Autodesk Inventor part; units mm, degrees
sketch "Sketch1" plane through (0, 0, 0) normal (0, 0, 1) x (1, 0, 0)
  line L0 (0, 0) -> (34, 0)
  line L1 (34, 0) -> (34, 4)
  line L2 (34, 4) -> (4, 4)
  line L3 (4, 4) -> (4, 154)
  line L4 (4, 154) -> (0, 154)
  line L5 (0, 154) -> (0, 0)
  dimension "d2" = 34
  dimension "d3" = 4
  dimension "d4" = 30
  dimension "d5" = 150
  dimension "d6" = 4
extrude "Extrusion1" add sketch "Sketch1" along normal blind 34
sketch "Sketch3" plane through (4, 4, 0) normal (1, 0, 0) x (0, 0, -1)
  line L0 (0, 0) -> (-34, 0)
  line L1 (0, 150) -> (-34, 150)
  arc A0 (-27, 20) -> (-7, 20) centre (-17, 20) ccw
  arc A1 (-7, 130) -> (-27, 130) centre (-17, 130) ccw
  line L2 (-27, 20) -> (-27, 130)
  line L3 (-7, 130) -> (-7, 20)
  point P0 (0, -4)
extrude "Extrusion3" cut sketch "Sketch3" against normal blind 20
sketch "Sketch4" plane through (0, 0, 0) normal (0, -1, 0) x (1, 0, 0)
  line L0 (0, 0) -> (34, 0)
  line L1 (34, 0) -> (34, 34)
  line L2 (0, 34) -> (34, 34)
  line L3 (0, 0) -> (0, 34)
  line L4 (4, 34) -> (0, 34)
  line L5 (34, 0) -> (34, 34)
  circle A0 centre (26.9999, 26.9999) radius 1.5
  circle A1 centre (26.9999, 7.0001) radius 1.5
  circle A2 centre (7.0001, 26.9999) radius 1.5
  circle A3 centre (7.0001, 7.0001) radius 1.5
  dimension "d28" = 3
  dimension "d29" = 3
  dimension "d30" = 3
  dimension "d31" = 3
extrude "Extrusion4" cut sketch "Sketch4" against normal blind 10 contours A0 | A1 | A2 | A3
sketch "Sketch5" plane through (4, 4, 0) normal (0, 1, 0) x (1, 0, 0)
  line L0 (0, 0) -> (0, -34)
  line L1 (36.8, 0) -> (-10.8, 0)
  line L2 (30, 0) -> (0, 0)
  line L3 (0, 0) -> (0, -2)
  line L4 (0, 0) -> (0, -34)
  line L5 (0, -2) -> (5, -2)
  line L6 (5, -2) -> (5, 0)
  line L7 (30, -34) -> (0, -34)
  line L8 (0, -34) -> (0, -32)
  line L9 (0, -32) -> (5, -32)
  line L10 (5, -32) -> (5, -34)
  line L11 (5, -34) -> (0, -34)
  point P0 (-4, 0)
  dimension "d34" = 2
  dimension "d35" = 5
  dimension "d36" = 2
  dimension "d37" = 5
extrude "Extrusion5" add sketch "Sketch5" along normal blind 5
sketch "Sketch6" plane through (0, 0, 0) normal (0, 0, -1) x (-1, 0, 0)
  line L0 (-34, 0) -> (-34, 4)
  line L1 (0, 0) -> (-34, 0)
  line L2 (0, 154) -> (0, 0)
  line L3 (-4, 154) -> (0, 154)
  line L4 (-4, 9) -> (-4, 154)
  line L5 (-9, 9) -> (-4, 9)
  line L6 (-9, 4) -> (-9, 9)
  line L7 (-34, 4) -> (-9, 4)
  line L8 (-4, 9) -> (-4, 4)
  line L9 (-9, 4) -> (-4, 9)
  line L10 (-4, 9) -> (-9, 9)
  line L11 (-4, 9) -> (-9, 9)
  line L12 (-9, 4) -> (-9, 9)
  line L13 (-9, 9) -> (-9, 4)
extrude "Extrusion6" cut sketch "Sketch6" against normal blind 4000 contours L6 L5 L9
properties part number "IDOM_infrared_fixture2"
CAD build for the part. Positions are in the model's coordinates, mm. A direction names the side the tool comes from. Round coordinates to 2 decimals unless told otherwise and drop trailing zeros. Write each loop counter-clockwise with the first axis right and the second up, starting at its lowest first coordinate (ties: lowest second). Pieces come first, ordered by that corner, then holes. Notation, with made-up numbers: (71.5, 11) -> (108.5, 11) arc R11 ccw to (108.5, 19) -> close; hole circle Ø1 at (73, 84.25). An arc over 180 degrees is marked (long way). Answer in a Markdown table with one row per item. Add a question column.
Item 1: Saw through at D-D, the plane x = 10.5. Write the cut outline in (y, z), then the cut area to 3 significant figures.
Item 2: Saw through at C-C, the plane z = 23. Write the cut outline in (x, y).
Item 3: Drop flat-ended pins along their axis: pin 1 Ø3.5 at (x, z) = (27, 7) entering from +Y; pin 2 Ø2.5 at (x, y) = (7.5, 7.5) entering from +Z; pin 3 Ø10 at (x, y) = (8, 86) entering from +Z. Give the stop position or say it passes through.
Item 4: Which spindle directions (+Z, -Z, +X, -X, +Y, -Y) get a long thin tool onto all of the face, cutting with end or side? Do faces 1 (the face through (7.806, 1.972, 8.265)), 2 (the face through (2, 78, 27)). Say none if no direction does.
Item 5: Saw through at B-B, the plane y = 87.5. Write the cut outline in (x, z), then the cut area to 3 significant figures.
Item 6: Mould opens along X. For faces 3 (the face through (6, 6, 2)), 4 (the face through (7.806, 1.972, 28.265)), 5 (the face through (4, 78, 28)) say: pulls with the +X half, pulls with the -X half, needs draft (parallel to the pull), parting line crosses it, or undercut.
Item 7: Saw through at A-A, the plane z = 17. Write the cut outline in (x, y), then the cut area to 3 significant figures.
Item 8: Drill centre lines: line 1 (Y direction, x = 23, z = 3); line 2 (Z direction, x = 2, y = 57). Where is each one in solid material? Low to high. Write a range as from..to.
Findings below:
| question | item | result |
|---|---|---|
| 1 | outline | (0, 0) -> (4, 0) -> (4, 34) -> (0, 34) -> close |
| 1 | area | 136 mm^2 |
| 2 | outline | (0, 0) -> (34, 0) -> (34, 4) -> (4, 4) -> (4, 16) -> (0, 16) -> close; (0, 142) -> (4, 142) -> (4, 154) -> (0, 154) -> close |
| 3 | pin 1 | stops at y = 4 |
| 3 | pin 2 | passes through |
| 3 | pin 3 | stops at z = 34 |
| 4 | face 1 | +Y, -Y |
| 4 | face 2 | +X, -X |
| 5 | outline | (0, 0) -> (4, 0) -> (4, 7) -> (0, 7) -> close; (0, 27) -> (4, 27) -> (4, 34) -> (0, 34) -> close |
| 5 | area | 56.0 mm^2 |
| 6 | face 3 | needs draft |
| 6 | face 4 | undercut |
| 6 | face 5 | pulls with the +X half |
| 7 | outline | (0, 0) -> (34, 0) -> (34, 4) -> (4, 4) -> (4, 14) -> (0, 14) -> close; (0, 144) -> (4, 144) -> (4, 154) -> (0, 154) -> close |
| 7 | area | 216 mm^2 |
| 8 | line 1 | y = 0..4 |
| 8 | line 2 | z = 0..7, 27..34 |
